Verification items for the finished model (mm, model axes). A direction names the side the tool comes from. Coordinates: 2 decimals unless noted, no trailing zeros. Order: outer loops, then holes, each group sorted by start corner. A loop starts at its lowest first (then second) coordinate and runs counter-clockwise, first axis right, second up. Notation, with made-up numbers: (12, -2.75) - (32, -2.75) arc R15 cw to (32, 23.25) - close; hole circle Ø7 at (36.5, 85). An arc over 180 degrees is marked (long way). One line per question, with ' | ' between items. Start each with the question number.
from build123d import *

# Parameters (mm, degrees)
BODY_DEPTH                           = 38.1
F_13_64_0_20313_DIAMETER_HOLE1_D     = 5.159502
F_13_64_0_20313_DIAMETER_HOLE1_DEPTH = 3.556
F_13_64_0_20313_DIAMETER_HOLE1_TIP   = 1.550070783
CHAMFER1_SIZE                        = 0.635
CHAMFER1_SIZE2                       = 0.366617421
CHAMFER1_PART_2_SIZE                 = 0.635
CHAMFER1_PART_2_SIZE2                = 0.366617421


with BuildPart() as part:
    # Profile → Body (new body)
    with BuildSketch(Plane(origin=(0, 0, 0), x_dir=(0, 0, -1), z_dir=(1, 0, 0))):
        Polygon((20, 1.905), (-20, 1.905), (-23.81, -1.905), (-27.62, -5.715), (-35.24, -13.335), (-40.32, -18.415), (-24.612052944, -18.415), (-21.679113577, -13.335), (-17.279704526, -5.715), (-15.08, -1.905), (-14.6, -1.905), (-5.4, -1.905), (-4.92, -1.905), (-2.720295474, -5.715), (-2.720295474, -13.335), (-2.720295474, -18.415), (2.720295474, -18.415), (2.720295474, -13.335), (2.720295474, -5.715), (4.92, -1.905), (5.4, -1.905), (14.6, -1.905), (15.08, -1.905), (17.279704526, -5.715), (21.679113577, -13.335), (24.612052944, -18.415), (40.32, -18.415), (35.24, -13.335), (27.62, -5.715), (23.81, -1.905), align=None)
    extrude(amount=BODY_DEPTH)

    # 13/64 (0.20313) Diameter Hole1
    with Locations(Plane(origin=(0, -1.905, 0), x_dir=(-1, 0, 0), z_dir=(0, -1, 0))):
        with Locations((-9.525, 10), (-9.525, -10), (-28.575, -10), (-28.575, 10)):
            Hole(F_13_64_0_20313_DIAMETER_HOLE1_D / 2, depth=F_13_64_0_20313_DIAMETER_HOLE1_DEPTH)
            with Locations((0, 0, -(F_13_64_0_20313_DIAMETER_HOLE1_DEPTH + F_13_64_0_20313_DIAMETER_HOLE1_TIP / 2))):  # 118° drill point
                Cone(0, F_13_64_0_20313_DIAMETER_HOLE1_D / 2, F_13_64_0_20313_DIAMETER_HOLE1_TIP, mode=Mode.SUBTRACT)

    # Chamfer1
    chamfer1_edges = [part.edges().sort_by_distance(p)[0] for p in [
        (25.995249, -1.905, -10),
        (6.945249, -1.905, -10),
    ]]
    chamfer1_side = [part.faces().sort_by_distance(p)[0] for p in [
        (19.05, -1.905, -10),
    ]]
    chamfer(chamfer1_edges, length=CHAMFER1_SIZE, length2=CHAMFER1_SIZE2, reference=chamfer1_side[0])

    # Chamfer1 part 2
    chamfer1_part_2_edges = [part.edges().sort_by_distance(p)[0] for p in [
        (25.995249, -1.905, 10),
        (6.945249, -1.905, 10),
    ]]
    chamfer1_part_2_side = [part.faces().sort_by_distance(p)[0] for p in [
        (19.05, -1.905, 10),
    ]]
    chamfer(chamfer1_part_2_edges, length=CHAMFER1_PART_2_SIZE, length2=CHAMFER1_PART_2_SIZE2, reference=chamfer1_part_2_side[0])


solid = part.part
Item 1: Thickness scan on probe 1 along X at (y, z) = (-0.3, -10); probe 2 along Z at (x, y) = (21, -17) (3 decimals); probe 3 along Z at (x, y) = (36, -16) (3 decimals). Record the ranges inside material, lowest first. Write a range as from..to.
Item 2: Gauge pin test, flat ends, axial feed: pin 1 (1 mm diameter, centred on x = 11, z = -5.5, fed in from -Y) (3 decimals); pin 2 (1.5 mm diameter, centred on x = 23.5, y = -15.5, fed in from -Z) (3 decimals); pin 3 (6.5 mm diameter, centred on x = 15, y = -10, fed in from -Z) (3 decimals); pin 4 (2 mm diameter, centred on y = -6, z = 4.5, fed in from +X). Record the tip position at first contact, or that the pin passes through.
Item 3: Section check C-C (z = 10). Record the cut outline in (x, y) (3 decimals), then the cut area to 3 significant figures.
Item 4: Section check A-A (y = -3). Record the cut outline in (x, z) (3 decimals).
Item 5: Set-up check for faces 1 (the flat face through (19, -18.415, 33)), 2 (the cylindrical face through (7.62, 0.08, 8.26)), 3 (the flat face through (18.783, -3.837, -3.805)): record each of +Z, -Z, +X, -X, +Y, -Y from which the full face is reachable in a straight line by a thin tool's end or side.
Item 6: Section check D-D (y = -11.25). Record the cut outline in (x, z) (3 decimals).
Item 7: Section check B-B (x = 4). Record the cut outline in (y, z) (3 decimals), then the cut area to 3 significant figures.
Item 8: Mould release check, pull along Z, two halves, no side actions. Record for faces 4 (the flat face through (19, 1.905, 0)), 5 (the cylindrical face through (7.62, 0.08, -11.74)), 6 (the flat face through (18.783, -3.783, 3.836)), 7 (the flat face through (18.783, -8.397, -30.302)): +Z half, -Z half, draft (parallel to the pull), parting line (faces both ways), or undercut.
Completed:
1) probe 1: x = 0..6.95, 12.1..26, 31.15..38.1 | probe 2: z = -38.905..-23.795, -2.72..2.72, 23.795..38.905 | probe 3: z = -37.905..-23.218, -2.72..2.72, 23.218..37.905
2) pin 1: stops at y = -1.905 | pin 2: stops at z = -38.155 | pin 3: stops at z = -35.155 | pin 4: passes through
3) outline: (0, -1.905) - (6.31, -1.905) - (6.945, -1.538) - (6.945, 1.651) - (7.368, 1.905) - (0, 1.905) - close; (11.682, 1.905) - (12.105, 1.651) - (12.105, -1.538) - (12.74, -1.905) - (25.36, -1.905) - (25.995, -1.538) - (25.995, 1.651) - (26.418, 1.905) - close; (30.732, 1.905) - (31.155, 1.651) - (31.155, -1.538) - (31.79, -1.905) - (38.1, -1.905) - (38.1, 1.905) - close | area: 106 mm^2
4) outline: (0, -24.905) - (38.1, -24.905) - (38.1, -15.712) - (0, -15.712) - close; (0, -4.288) - (38.1, -4.288) - (38.1, 4.288) - (0, 4.288) - close; (0, 15.712) - (38.1, 15.712) - (38.1, 24.905) - (0, 24.905) - close
5) face 1: +Z, -Z, +X, -X, -Y | face 2: -Y | face 3: +X, -X, -Y
6) outline: (0, -33.155) - (38.1, -33.155) - (38.1, -20.475) - (0, -20.475) - close; (0, -2.72) - (38.1, -2.72) - (38.1, 2.72) - (0, 2.72) - close; (0, 20.475) - (38.1, 20.475) - (38.1, 33.155) - (0, 33.155) - close
7) outline: (-18.415, -40.32) - (1.905, -20) - (1.905, 20) - (-18.415, 40.32) - (-18.415, 24.612) - (-1.905, 15.08) - (-1.905, 4.92) - (-5.715, 2.72) - (-18.415, 2.72) - (-18.415, -2.72) - (-5.715, -2.72) - (-1.905, -4.92) - (-1.905, -15.08) - (-18.415, -24.612) - close | area: 669 mm^2
8) face 4: draft | face 5: undercut | face 6: undercut | face 7: -Z half
